Autodesk Inventor part; units mm, degrees
ref_plane "YZ Plane" through (0, 0, 0) normal (1, 0, 0) x (0, 1, 0)
ref_plane "XZ Plane" through (0, 0, 0) normal (0, 1, 0) x (-1, 0, 0)
ref_plane "XY Plane" through (0, 0, 0) normal (0, 0, 1) x (1, 0, 0)
sketch "Sketch1" plane through (0, 0, 0) normal (0, 0, 1) x (1, 0, 0)
  line L0 (22.975, -85.9934) -> (22.975, 16.5133)
  line L1 (22.975, 16.5133) -> (13.1755, 28.0421)
  arc A0 (13.1755, 28.0421) -> (12.4, 28.6015) centre (11.6516, 26.7468) ccw
  arc A1 (-12.4, 28.6015) -> (-13.1755, 28.0421) centre (-11.6516, 26.7468) ccw
  line L2 (-13.1755, 28.0421) -> (-22.975, 16.5133)
  line L3 (-22.975, 16.5133) -> (-22.975, -85.4265)
  line L4 (-12.975, -95.4265) -> (-22.975, -85.4265)
  line L5 (-12.975, -95.4265) -> (13.594, -95.4265)
  line L6 (22.975, -85.9934) -> (13.594, -95.4265)
  line L7 (-6, -127.9265) -> (-8.9861, -127.9265)
  arc A2 (-6, -127.9265) -> (-4, -125.9265) centre (-6, -125.9265) ccw
  line L8 (-4, -125.9265) -> (-4, -125.4265)
  arc A3 (4, -125.4265) -> (-4, -125.4265) centre (0, -125.4265) ccw
  line L9 (4, -125.9265) -> (4, -125.4265)
  arc A4 (4, -125.9265) -> (6, -127.9265) centre (6, -125.9265) ccw
  line L10 (8.9861, -127.9265) -> (6, -127.9265)
  arc A5 (8.9861, -127.9265) -> (10.983, -126.0376) centre (8.9861, -125.9265) ccw
  arc A6 (10.983, -126.0376) -> (11, -125.4265) centre (0, -125.4265) ccw
  line L11 (11, -125.4265) -> (11, -96.9265)
  line L12 (-11, -125.4265) -> (-11, -96.9265)
  arc A7 (-11, -125.4265) -> (-10.983, -126.0376) centre (0, -125.4265) ccw
  arc A8 (-10.983, -126.0376) -> (-8.9861, -127.9265) centre (-8.9861, -125.9265) ccw
  line L13 (-11, -96.9265) -> (-11, -95.4265)
  line L14 (11, -96.9265) -> (11, -95.4265)
  line L15 (-12.4, 28.6015) -> (12.4, 28.6015)
  circle A9 centre (0, 16.6015) radius 11
  dimension "d0" = 22
extrude "Extrusion1" add sketch "Sketch1" along normal mid plane 36 contours L6 L5 L4 L3 L2 A1 L15 A0 L1 L0
extrude "Extrusion2" add sketch "Sketch1" along normal mid plane 41 contours A9
sketch "Sketch2" plane through (-12.975, -95.4265, 18) normal (0, -1, 0) x (1, 0, 0)
  line L0 (1.975, 4) -> (23.975, 4)
  line L1 (23.975, 4) -> (23.975, -40)
  line L2 (23.975, -40) -> (1.975, -40)
  line L3 (1.975, -40) -> (1.975, 4)
  point P0 (12.975, -18)
  point P1 (12.975, -18)
  point P2 (12.975, -18)
  dimension "d5" = 22
  dimension "d6" = 44
  dimension "d16" = 22
extrude "Extrusion3" add sketch "Sketch2" along normal blind 1.5
sketch "Sketch3" plane through (-12.975, -96.9265, 18) normal (0, -1, 0) x (1, 0, 0)
  line L0 (23.975, 4) -> (23.975, -40)
  line L1 (1.975, -40) -> (1.975, 4)
  line L2 (1.975, 4) -> (23.975, 4)
  line L3 (23.975, 4) -> (23.975, 2.5)
  line L4 (23.975, 2.5) -> (1.975, 2.5)
  line L5 (1.975, 2.5) -> (1.975, 4)
  line L6 (23.975, -40) -> (1.975, -40)
  line L7 (1.975, -40) -> (1.975, -38.5)
  line L8 (1.975, -38.5) -> (23.975, -38.5)
  line L9 (23.975, -38.5) -> (23.975, -40)
  point P0 (12.975, -18)
  dimension "d9" = 1.5
  dimension "d10" = 1.5
extrude "Extrusion4" add sketch "Sketch3" along normal blind 32 contours L0 L4 L1 L2 | L0 L6 L1 L8
sketch "Sketch4" plane through (11, -95.4265, -22) normal (0, 0, -1) x (-1, 0, 0)
  line L0 (22, 0) -> (22, -33.5)
  line L1 (0, 0) -> (22, 0)
  line L2 (0, 0) -> (0, -33.5)
  line L3 (0, -33.5) -> (22, -33.5)
  arc A0 (15, -30) -> (7, -30) centre (11, -30) ccw
  arc A1 (5, -32.5) -> (7, -30.5) centre (5, -30.5) ccw
  line L4 (2.0139, -32.5) -> (5, -32.5)
  line L5 (15, -30.5) -> (15, -30)
  line L6 (7, -30.5) -> (7, -30)
  arc A2 (0.017, -30.6111) -> (2.0139, -32.5) centre (2.0139, -30.5) ccw
  line L7 (17, -32.5) -> (19.9861, -32.5)
  arc A3 (15, -30.5) -> (17, -32.5) centre (17, -30.5) ccw
  arc A4 (19.9861, -32.5) -> (21.983, -30.6111) centre (19.9861, -30.5) ccw
  arc A5 (21.983, -30.6111) -> (22, -30) centre (11, -30) ccw
  arc A6 (0, -30) -> (0.017, -30.6111) centre (11, -30) ccw
  point P0 (11, 95.4265)
extrude "Extrusion5" cut sketch "Sketch4" against normal through all contours L0 L3 L2 A6 A2 L4 A1 L6 A0 L5 A3 L7 A4 A5
properties part number "ForeArm"
The listing builds one solid part. Answer for the finished solid, in the listing's coordinates (mm). A direction names the side the tool comes from. Round coordinates to 2 decimals unless told otherwise and drop trailing zeros. Order: outer loops, then holes, each group sorted by start corner. A loop starts at its lowest first (then second) coordinate and runs counter-clockwise, first axis right, second up. Notation, with made-up numbers: (-20, -25) -> (30, -25) arc R22 cw to (30, -17) -> close; hole circle Ø3 at (51.5, 26.25). An arc over 180 degrees is marked (long way). Answer as CSV lines item,"result". Start each with the question number.
(1) The part is cut by section B-B (z = 2). Determine the outline of the cut face in (x, y) (1 decimal), then the cut area to 3 significant figures.
(2) The part is cut by section C-C (x = 0). Determine the outline of the cut face in (y, z).
(3) Flat-ended cylindrical pins translate along their axes: pin 1 Ø1.2 at (x, z) = (5, 20) entering from +Y; pin 2 Ø0.6 at (y, z) = (-125.5, -21) entering from +X; pin 3 Ø17.5 at (x, y) = (-0.5, 13) entering from -Z; pin 4 Ø9 at (y, z) = (-103.5, -10) entering from -X. Find the tip coordinate at first contact, or state that the pin passes through.
(4) The part is cut by section A-A (y = -107). Determine the outline of the cut face in (x, z).
(5) For a pull along X with two mould halves and no side action, classify faces 1 (the face through (0, -33, 18)), 2 (the face through (22.975, -35, 0)), 3 (the face through (-0.088, -121.427, -21.26)) as +X half, -X half, draft (parallel to the pull), parting line (faces both ways), or undercut.
(6) A tool of negligible diameter and unlimited length cuts with its end or side. For faces 4 (the face through (-2.385, 5.863, -19.232)), 5 (the face through (0, -112, -20.5)), 6 (the face through (0, -95.426, 20)), from which of +Z, -Z, +X, -X, +Y, -Y can it reach the whole face along a straight path? Write none if from no direction.
(7) The part is cut by section D-D (y = -44). Determine the outline of the cut face in (x, z) (3 decimals).
(8) Find the intervals of material crossed by probe 1 along Z at (x, y) = (-8, -121); probe 2 along Z at (x, y) = (-8, -27.5); probe 3 along Y at (x, z) = (0, -13), in increasing order. Write a range as from..to.
Evaluation:
1,outline,"(-23, -85.4) -> (-13, -95.4) -> (-11, -95.4) -> (-11, -96.9) -> (11, -96.9) -> (11, -95.4) -> (13.6, -95.4) -> (23, -86) -> (23, 16.5) -> (13.2, 28) arc R2 ccw to (12.4, 28.6) -> (-12.4, 28.6) arc R2 ccw to (-13.2, 28) -> (-23, 16.5) -> close"
1,area,"5,510 mm²"
2,outline,"(-121.43, -22) -> (-95.43, -22) -> (-95.43, -18) -> (5.6, -18) -> (5.6, -20.5) -> (27.6, -20.5) -> (27.6, -18) -> (28.6, -18) -> (28.6, 18) -> (27.6, 18) -> (27.6, 20.5) -> (5.6, 20.5) -> (5.6, 18) -> (-95.43, 18) -> (-95.43, 22) -> (-121.43, 22) -> (-121.43, 20.5) -> (-96.93, 20.5) -> (-96.93, -20.5) -> (-121.43, -20.5) -> close"
3,pin 1,"y = 26.68"
3,pin 2,"x = 11"
3,pin 3,"z = -20.5"
3,pin 4,"through"
4,outline,"(-11, -22) -> (11, -22) -> (11, -20.5) -> (-11, -20.5) -> close; (-11, 20.5) -> (11, 20.5) -> (11, 22) -> (-11, 22) -> close"
5,face 1,"draft"
5,face 2,"+X half"
5,face 3,"undercut"
6,face 4,"-Z"
6,face 5,"+X, -X, -Y"
6,face 6,"+Z, +X, -X"
7,outline,"(-22.975, -18) -> (22.975, -18) -> (22.975, 18) -> (-22.975, 18) -> close"
8,probe 1,"-22..-20.5, 20.5..22"
8,probe 2,"-18..18"
8,probe 3,"-96.93..28.6"
